```python
from build123d import *

# Parameters (mm, degrees)
SKETCH2_W                = 200
SKETCH2_H                = 150
BOSS_EXTRUDE1_DEPTH      = 80
FILLET1_R                = 10
SHELL1_T                 = -2
SHELL1_THICKNESS_2_DEPTH = 13
SKETCH5_W                = 36.5
SKETCH5_H                = 27.5
CUT_EXTRUDE1_DEPTH       = 2
BOSS_EXTRUDE2_DEPTH      = 16
SKETCH7_W                = 36.5
SKETCH7_H                = 27.5
CUT_EXTRUDE2_DEPTH       = 2
BOSS_EXTRUDE3_DEPTH      = 16
SKETCH10_W               = 36.5
SKETCH10_H               = 27.5
CUT_EXTRUDE4_DEPTH       = 2
BOSS_EXTRUDE4_DEPTH      = 16
SKETCH13_W               = 38
SKETCH13_H               = 19.1
CUT_EXTRUDE5_DEPTH       = 2
BOSS_EXTRUDE5_DEPTH      = 13.5
SKETCH15_W               = 10.5
SKETCH15_H               = 9.367949192
CUT_EXTRUDE6_DEPTH       = 3
CUT_EXTRUDE8_REACH       = 150.408
SKETCH20_R               = 8
SPLIT1_SURFACE_1_BACK    = 263.488
SPLIT1_SURFACE_1_DEPTH   = 526.976
SPLIT1_SURFACE_2_BACK    = 263.488
SPLIT1_SURFACE_2_DEPTH   = 526.976
SPLIT2_SURFACE_3_BACK    = 263.488
SPLIT2_SURFACE_3_DEPTH   = 526.976
SPLIT2_SURFACE_4_BACK    = 263.488
SPLIT2_SURFACE_4_DEPTH   = 526.976


with BuildPart() as part:
    # Sketch2 → Boss-Extrude1 (new body)
    with BuildSketch(Plane(origin=(0, 0, 0), x_dir=(1, 0, 0), z_dir=(0, 1, 0))):
        Rectangle(SKETCH2_W, SKETCH2_H)
    extrude(amount=BOSS_EXTRUDE1_DEPTH)

    # Fillet1
    fillet1_edges = [part.edges().sort_by_distance(p)[0] for p in [
        (100, 40, 75),
        (-100, 40, 75),
        (-100, 40, -75),
        (100, 40, -75),
    ]]
    fillet(fillet1_edges, radius=FILLET1_R)

    # Shell1
    shell1_openings = [part.faces().sort_by_distance(p)[0] for p in [
        (0, 80, 0),
    ]]
    offset(amount=SHELL1_T, openings=shell1_openings, kind=Kind.INTERSECTION)

    # Shell1 thickness 2 face (on inner face of the shell) → Shell1 thickness 2 (add)
    with BuildSketch(Plane(origin=(0, 2, 0), x_dir=(0, 0, -1), z_dir=(0, -1, 0))):
        with BuildLine():
            ThreePointArc((73, -90), (70.656854249, -95.656854249), (65, -98))
            Line((65, -98), (-65, -98))
            ThreePointArc((-65, -98), (-70.656854249, -95.656854249), (-73, -90))
            Line((-73, -90), (-73, 90))
            ThreePointArc((-73, 90), (-70.656854249, 95.656854249), (-65, 98))
            Line((-65, 98), (65, 98))
            ThreePointArc((65, 98), (70.656854249, 95.656854249), (73, 90))
            Line((73, 90), (73, -90))
        make_face()
    extrude(amount=-SHELL1_THICKNESS_2_DEPTH)

    # Sketch5 → Cut-Extrude1 (cut)
    with BuildSketch(Plane.XY.offset(75)):
        with Locations((0, 30.75)):
            Rectangle(SKETCH5_W, SKETCH5_H)
        Polygon((-18.25, 43.5), (-19.75, 44.366025404), (-19.75, 41.633974596), (-18.25, 42.5), align=None)
        Polygon((-19.75, 19.866025404), (-18.25, 19), (-18.25, 18), (-19.75, 17.133974596), align=None)
        Polygon((19.75, 17.133974596), (19.75, 19.866025404), (18.25, 19), (18.25, 18), align=None)
        Polygon((19.75, 41.633974596), (18.25, 42.5), (18.25, 43.5), (19.75, 44.366025404), align=None)
    extrude(amount=-CUT_EXTRUDE1_DEPTH, mode=Mode.SUBTRACT)

    # Sketch6 → Boss-Extrude2 (add)
    with BuildSketch(Plane(origin=(0, 0, 73), x_dir=(-1, 0, 0), z_dir=(0, 0, -1))):
        Polygon((18.25, 15), (21.25, 15), (21.25, 47.5), (18.25, 47.5), (18.25, 43.5), (19.75, 44.366025404), (19.75, 41.633974596), (18.25, 42.5), (18.25, 19), (19.75, 19.866025404), (19.75, 17.133974596), (18.25, 18), align=None)
        Polygon((-21.25, 47.5), (-21.25, 15), (-18.25, 15), (-18.25, 18), (-19.75, 17.133974596), (-19.75, 19.866025404), (-18.25, 19), (-18.25, 42.5), (-19.75, 41.633974596), (-19.75, 44.366025404), (-18.25, 43.5), (-18.25, 47.5), align=None)
    extrude(amount=BOSS_EXTRUDE2_DEPTH)

    # Sketch7 → Cut-Extrude2 (cut)
    with BuildSketch(Plane(origin=(100, 0, 0), x_dir=(0, 0, -1), z_dir=(1, 0, 0))):
        with Locations((0, 30.75)):
            Rectangle(SKETCH7_W, SKETCH7_H)
        Polygon((-18.25, 43.5), (-19.75, 44.366025404), (-19.75, 41.633974596), (-18.25, 42.5), align=None)
        Polygon((-19.75, 19.866025404), (-18.25, 19), (-18.25, 18), (-19.75, 17.133974596), align=None)
        Polygon((19.75, 17.133974596), (19.75, 19.866025404), (18.25, 19), (18.25, 18), align=None)
        Polygon((19.75, 41.633974596), (18.25, 42.5), (18.25, 43.5), (19.75, 44.366025404), align=None)
    extrude(amount=-CUT_EXTRUDE2_DEPTH, mode=Mode.SUBTRACT)

    # Sketch8 → Boss-Extrude3 (add)
    with BuildSketch(Plane.ZY.offset(-98)):
        Polygon((-21.25, 47.5), (-18.25, 47.5), (-18.25, 43.5), (-19.75, 44.366025404), (-19.75, 41.633974596), (-18.25, 42.5), (-18.25, 19), (-19.75, 19.866025404), (-19.75, 17.133974596), (-18.25, 18), (-18.25, 15), (-21.25, 15), align=None)
        Polygon((19.75, 44.366025404), (18.25, 43.5), (18.25, 47.5), (21.25, 47.5), (21.25, 15), (18.25, 15), (18.25, 18), (19.75, 17.133974596), (19.75, 19.866025404), (18.25, 19), (18.25, 42.5), (19.75, 41.633974596), align=None)
    extrude(amount=BOSS_EXTRUDE3_DEPTH)

    # Sketch10 → Cut-Extrude4 (cut)
    with BuildSketch(Plane.ZY.offset(100)):
        with Locations((0, 30.75)):
            Rectangle(SKETCH10_W, SKETCH10_H)
        Polygon((-18.25, 43.5), (-19.75, 44.366025404), (-19.75, 41.633974596), (-18.25, 42.5), align=None)
        Polygon((-19.75, 19.866025404), (-18.25, 19), (-18.25, 18), (-19.75, 17.133974596), align=None)
        Polygon((19.75, 17.133974596), (19.75, 19.866025404), (18.25, 19), (18.25, 18), align=None)
        Polygon((19.75, 41.633974596), (18.25, 42.5), (18.25, 43.5), (19.75, 44.366025404), align=None)
    extrude(amount=-CUT_EXTRUDE4_DEPTH, mode=Mode.SUBTRACT)

    # Sketch11 → Boss-Extrude4 (add)
    with BuildSketch(Plane(origin=(-98, 0, 0), x_dir=(0, 0, -1), z_dir=(1, 0, 0))):
        Polygon((-18.25, 47.5), (-21.25, 47.5), (-21.25, 15), (-18.25, 15), (-18.25, 18), (-19.75, 17.133974596), (-19.75, 19.866025404), (-18.25, 19), (-18.25, 42.5), (-19.75, 41.633974596), (-19.75, 44.366025404), (-18.25, 43.5), align=None)
        Polygon((19.75, 44.366025404), (18.25, 43.5), (18.25, 47.5), (21.25, 47.5), (21.25, 15), (18.25, 15), (18.25, 18), (19.75, 17.133974596), (19.75, 19.866025404), (18.25, 19), (18.25, 42.5), (19.75, 41.633974596), align=None)
    extrude(amount=BOSS_EXTRUDE4_DEPTH)

    # Sketch13 → Cut-Extrude5 (cut)
    with BuildSketch(Plane.XY.offset(75)):
        Polygon((41, 39.3), (39.5, 40.166025404), (39.5, 37.433974596), (41, 38.3), align=None)
        with Locations((60, 30.75)):
            Rectangle(SKETCH13_W, SKETCH13_H)
        Polygon((41, 22.2), (39.5, 21.333974596), (39.5, 24.066025404), (41, 23.2), align=None)
        Polygon((79, 22.2), (79, 23.2), (80.5, 24.066025404), (80.5, 21.333974596), align=None)
        Polygon((79, 39.3), (80.5, 40.166025404), (80.5, 37.433974596), (79, 38.3), align=None)
    extrude(amount=-CUT_EXTRUDE5_DEPTH, mode=Mode.SUBTRACT)

    # Sketch14 → Boss-Extrude5 (add)
    with BuildSketch(Plane(origin=(0, 0, 73), x_dir=(-1, 0, 0), z_dir=(0, 0, -1))):
        Polygon((-79, 43.3), (-82, 43.3), (-82, 15), (-79, 15), (-79, 22.2), (-80.5, 21.333974596), (-80.5, 24.066025404), (-79, 23.2), (-79, 38.3), (-80.5, 37.433974596), (-80.5, 40.166025404), (-79, 39.3), align=None)
        Polygon((-39.5, 40.166025404), (-41, 39.3), (-41, 43.3), (-38, 43.3), (-38, 15), (-41, 15), (-41, 22.2), (-39.5, 21.333974596), (-39.5, 24.066025404), (-41, 23.2), (-41, 38.3), (-39.5, 37.433974596), align=None)
    extrude(amount=BOSS_EXTRUDE5_DEPTH)

    # Sketch15 → Cut-Extrude6 (cut)
    with BuildSketch(Plane.ZY.offset(-38)):
        with Locations((66.75, 30.75)):
            Rectangle(SKETCH15_W, SKETCH15_H)
    extrude(amount=-CUT_EXTRUDE6_DEPTH, mode=Mode.SUBTRACT)

    # Sketch18 → Cut-Revolve1 (revolve, cut)
    with BuildSketch(Plane(origin=(0, 0, 0), x_dir=(0, 0, -1), z_dir=(1, 0, 0)), mode=Mode.PRIVATE) as cut_revolve1_sk:
        Polygon((-42.5, 0), (-70, 0), (-47.5, 10), (-42.5, 10), align=None)
    revolve(cut_revolve1_sk.sketch.rotate(Axis((0, 0, 0), (0, 1, 0)), 180), axis=Axis((0, 0, 0), (0, 1, 0)), mode=Mode.SUBTRACT)

    # Cut-Extrude8: up to this face of the body (flat: up to its plane)
    cut_extrude8_end = Plane(part.part.faces().sort_by_distance((-0.172388952, 15, -0.411685035))[0])
    # Sketch20 → Cut-Extrude8 (cut, up to the picked face)
    with BuildSketch(Plane.XZ, mode=Mode.PRIVATE) as cut_extrude8_sk1:
        with Locations(Location((0, -42.5, 0), (0, 0, 270))):
            Circle(SKETCH20_R)
    cut_extrude8_tool1 = split(extrude(cut_extrude8_sk1.sketch, amount=-CUT_EXTRUDE8_REACH, mode=Mode.PRIVATE), bisect_by=cut_extrude8_end, keep=Keep.BOTH, mode=Mode.PRIVATE)
    add(cut_extrude8_tool1.solids().sort_by(Axis((0, 0, -42.5), (0, 1, 0)))[0], mode=Mode.SUBTRACT)


with BuildPart() as body_2:
    # Split1: the piece behind the surface
    add(part.part)
    # Split1 surface: a surface, the sketch's curves swept straight by 526.976 mm
    with BuildLine(Plane.XY.offset(75).offset(-SPLIT1_SURFACE_1_BACK), mode=Mode.PRIVATE) as split1_surface_1_path:
        Line((-23.25, 49.5), (23.25, 49.5))
        Line((23.25, 49.5), (23.25, 12))
        Line((23.25, 12), (-23.25, 12))
        Line((-23.25, 12), (-23.25, 49.5))
    split1_surface_1 = Shell.extrude(split1_surface_1_path.wire(), (0 * SPLIT1_SURFACE_1_DEPTH, 0 * SPLIT1_SURFACE_1_DEPTH, 1 * SPLIT1_SURFACE_1_DEPTH))
    split(bisect_by=split1_surface_1, keep=Keep.BOTTOM)


with BuildPart() as part_1:
    add(part.part)

    # Split1: split by a surface, the side it looks to stays
    # Split1 surface: a surface, the sketch's curves swept straight by 526.976 mm
    with BuildLine(Plane.XY.offset(75).offset(-SPLIT1_SURFACE_2_BACK), mode=Mode.PRIVATE) as split1_surface_2_path:
        Line((-23.25, 49.5), (23.25, 49.5))
        Line((23.25, 49.5), (23.25, 12))
        Line((23.25, 12), (-23.25, 12))
        Line((-23.25, 12), (-23.25, 49.5))
    split1_surface_2 = Shell.extrude(split1_surface_2_path.wire(), (0 * SPLIT1_SURFACE_2_DEPTH, 0 * SPLIT1_SURFACE_2_DEPTH, 1 * SPLIT1_SURFACE_2_DEPTH))
    split(bisect_by=split1_surface_2, keep=Keep.TOP)


with BuildPart() as body_3:
    # Split2: the piece behind the surface
    add(body_2.part)
    # Split2 surface: a surface, the sketch's curves swept straight by 526.976 mm
    with BuildLine(Plane(origin=(0, 15, 0), x_dir=(1, 0, 0), z_dir=(0, 1, 0)).offset(-SPLIT2_SURFACE_3_BACK), mode=Mode.PRIVATE) as split2_surface_3_path:
        Line((-23.25, -75), (23.25, -75))
        Line((23.25, -75), (23.25, -50))
        Line((23.25, -50), (-23.25, -50))
        Line((-23.25, -50), (-23.25, -75))
    split2_surface_3 = Shell.extrude(split2_surface_3_path.wire(), (0 * SPLIT2_SURFACE_3_DEPTH, 1 * SPLIT2_SURFACE_3_DEPTH, 0 * SPLIT2_SURFACE_3_DEPTH))
    split(bisect_by=split2_surface_3, keep=Keep.BOTTOM)


with BuildPart() as body_2_1:
    add(body_2.part)

    # Split2: split by a surface, the side it looks to stays
    # Split2 surface: a surface, the sketch's curves swept straight by 526.976 mm
    with BuildLine(Plane(origin=(0, 15, 0), x_dir=(1, 0, 0), z_dir=(0, 1, 0)).offset(-SPLIT2_SURFACE_4_BACK), mode=Mode.PRIVATE) as split2_surface_4_path:
        Line((-23.25, -75), (23.25, -75))
        Line((23.25, -75), (23.25, -50))
        Line((23.25, -50), (-23.25, -50))
        Line((-23.25, -50), (-23.25, -75))
    split2_surface_4 = Shell.extrude(split2_surface_4_path.wire(), (0 * SPLIT2_SURFACE_4_DEPTH, 1 * SPLIT2_SURFACE_4_DEPTH, 0 * SPLIT2_SURFACE_4_DEPTH))
    split(bisect_by=split2_surface_4, keep=Keep.TOP)


solid = body_2_1.part
```
Could you check a few things on this model? Use its own coordinates, in mm. A direction names the side the tool comes from. Coordinates: 2 decimals unless noted, no trailing zeros. Write each loop counter-clockwise with the first axis right and the second up, starting at its lowest first coordinate (ties: lowest second). Pieces come first, ordered by that corner, then holes. Notation, with made-up numbers: (35, -21.75) -> (57, -21.75) arc R13 ccw to (57, -3.75) -> close; hole circle Ø2 at (77.25, 10). An arc over 180 degrees is marked (long way). Write item = value, one per line. Start each with the question number.
(1) I need wall thicknesses on line 1 (X direction, y = 34, z = 63); line 2 (X direction, y = 19.5, z = 58.75); line 3 (Y direction, x = 18.5, z = 63.75). Which ranges of each line are inside material? Lowest first, please. Write a range as [from, to].
(2) I want a section at C-C (z = 58). Please give me the cut outline in (x, y).
(3) I want a section at A-A (x = 10.5). Please give me the cut outline in (y, z), plus the area to 3 significant figures.
(4) I want a section at B-B (y = 38). Please give me the cut outline in (x, z), plus the area to 3 significant figures.
(5) Which directions (+Z, -Z, +X, -X, +Y, -Y) give clear straight access to the entire face, cutting with the end or side of a thin tool? Please do faces 1 (the face through (19.75, 43, 66)), 2 (the face through (20, 31, 57)), 3 (the face through (0, 47, 75)).
(6) Will these pins go through, and if not, where does the flat tip stop? pin 1 (1 mm diameter, centred on x = 13, z = 66.5, fed in from +Y); pin 2 (1.4 mm diameter, centred on y = 19, z = 69.5, fed in from +X); pin 3 (2.5 mm diameter, centred on x = 20, z = 63, fed in from +Y); pin 4 (12 mm diameter, centred on x = -18, y = 37, fed in from +Z).
(7) We'd pull the mould along Y, two halves only. Please class faces 4 (the face through (19.01, 19.44, 66.13)), 5 (the face through (20, 47.5, 65)), 6 (the face through (0, 16, 73)): released by +Y, released by -Y, zero draft, split by the parting line, or undercut.
(8) I want a section at D-D (x = -19). Please give me the cut outline in (y, z).
Result set:
q1.line_1 = [-21.25, -18.25], [18.25, 21.25]
q1.line_2 = [-21.25, -19.75], [-19.12, -18.25], [18.25, 19.12], [19.75, 21.25]
q1.line_3 = [12, 17.86], [19.14, 42.36], [43.64, 47.5]
q2.outline = (-23.25, 12) -> (23.25, 12) -> (23.25, 15) -> (21.25, 15) -> (21.25, 47.5) -> (18.25, 47.5) -> (18.25, 43.5) -> (19.75, 44.37) -> (19.75, 41.63) -> (18.25, 42.5) -> (18.25, 19) -> (19.75, 19.87) -> (19.75, 17.13) -> (18.25, 18) -> (18.25, 15) -> (-18.25, 15) -> (-18.25, 18) -> (-19.75, 17.13) -> (-19.75, 19.87) -> (-18.25, 19) -> (-18.25, 42.5) -> (-19.75, 41.63) -> (-19.75, 44.37) -> (-18.25, 43.5) -> (-18.25, 47.5) -> (-21.25, 47.5) -> (-21.25, 15) -> (-23.25, 15) -> close
q3.outline = (12, 50) -> (15, 50) -> (15, 73) -> (17, 73) -> (17, 75) -> (12, 75) -> close; (44.5, 73) -> (49.5, 73) -> (49.5, 75) -> (44.5, 75) -> close
q3.area = 89.0 mm2
q4.outline = (-23.25, 73) -> (-21.25, 73) -> (-21.25, 57) -> (-18.25, 57) -> (-18.25, 75) -> (-23.25, 75) -> close; (18.25, 57) -> (21.25, 57) -> (21.25, 73) -> (23.25, 73) -> (23.25, 75) -> (18.25, 75) -> close
q4.area = 116 mm2
q5.face_1 = +Z, -Z
q5.face_2 = -Z, +X, -X, +Y
q5.face_3 = +Z, +X, -X, +Y, -Y
q6.pin_1 = 15
q6.pin_2 = 21.25
q6.pin_3 = 47.5
q6.pin_4 = 75
q7.face_4 = undercut
q7.face_5 = released by +Y
q7.face_6 = zero draft
q8.outline = (12, 50) -> (15, 50) -> (15, 57) -> (17.57, 57) -> (17.57, 75) -> (12, 75) -> close; (19.43, 57) -> (42.07, 57) -> (42.07, 75) -> (19.43, 75) -> close; (43.93, 57) -> (47.5, 57) -> (47.5, 73) -> (49.5, 73) -> (49.5, 75) -> (43.93, 75) -> close
